from build123d import *

# Parameters (mm, degrees)
SKETCH_W        = 3.9
SKETCH_H        = 9.9
PAD_DEPTH       = 1.4
POCKET_DEPTH    = 9.901
POCKET001_DEPTH = 3.901
POCKET002_DEPTH = 0.1


with BuildPart() as part:
    # Sketch → Pad (new body)
    with BuildSketch(Plane.XY):
        Rectangle(SKETCH_W, SKETCH_H)
    extrude(amount=PAD_DEPTH)

    # Sketch001 (on Face3 of Pad) → Pocket (cut, through all)
    with BuildSketch(Plane.XZ.offset(4.95)):
        Polygon((-1.95, 0.6), (-1.65, 0), (-1.95, 0), align=None)
        Polygon((1.65, 0), (1.95, 0), (1.95, 0.6), align=None)
        Polygon((1.95, 1.4), (1.65, 1.4), (1.95, 0.8), align=None)
        Polygon((-1.95, 1.4), (-1.65, 1.4), (-1.95, 0.8), align=None)
    extrude(amount=-POCKET_DEPTH, mode=Mode.SUBTRACT)

    # Sketch002 (on Face5 of Pocket) → Pocket001 (cut, through all)
    with BuildSketch(Plane.YZ.offset(1.95)):
        Polygon((4.95, 0.8), (4.65, 1.4), (4.95, 1.4), align=None)
        Polygon((4.95, 0.6), (4.65, 0), (4.95, 0), align=None)
        Polygon((-4.95, 0.8), (-4.95, 1.4), (-4.65, 1.4), align=None)
        Polygon((-4.95, 0.6), (-4.95, 0), (-4.65, 0), align=None)
    extrude(amount=-POCKET001_DEPTH, mode=Mode.SUBTRACT)

    # Sketch003 (on Face11 of Pocket001) → Pocket002 (cut)
    with BuildSketch(Plane.XY.offset(1.4)):
        with BuildLine():
            ThreePointArc((-0.429098, 4.124211), (0, 3.695113), (0.429098, 4.124211))
            Line((0.429098, 4.124211), (0.429098, 5.299881))
            ThreePointArc((0.429098, 5.299881), (0, 5.728979), (-0.429098, 5.299881))
            Line((-0.429098, 4.124211), (-0.429098, 5.299881))
        make_face()
    extrude(amount=-POCKET002_DEPTH, mode=Mode.SUBTRACT)


with BuildPart() as part_1:
    # Body placement: moved
    add(part.part.moved(Location((0, 0, 0.1))))


solid = part_1.part
Verification items for the finished model (mm, model axes). Give positions to 0.01 mm unless a question says otherwise; leave off trailing zeros. Write each loop counter-clockwise with the first axis right and the second up, starting at its lowest first coordinate (ties: lowest second). Pieces come first, ordered by that corner, then holes. Notation, with made-up numbers: (-29, -37.5) - (-1, -37.5) arc R15 ccw to (-1, -10.5) - close; hole circle Ø5 at (19, 9.5). An arc over 180 degrees is marked (long way). Answer as CSV lines item,"result". Start each with the question number.
1. Draft check along X on faces 1 (the face through (0, 0, 1.5)), 2 (the face through (0, 4, 1.4)). Enter one of: pulls with the +X half, pulls with the -X half, needs draft (parallel to the pull), parting line crosses it, or undercut.
2. Sectioned sample at D-D (x = 1.5). Record the boundary of the cut face in (y, z), then the cut area to 3 significant figures.
3. Thickness scan on line 1 (Y direction, x = 1.25, z = 0.55) (3 decimals); line 2 (Y direction, x = -1.25, z = 1.2); line 3 (X direction, y = 1, z = 0.35) (3 decimals). Record the ranges inside material, lowest first.
4. Depth check by flat-ended pin: pin 1 (0.7 mm diameter, centred on x = 0, y = 4.5, fed in from +Z). Enter the tip coordinate at first touch or a pass-through.
5. Sectioned sample at A-A (y = -0.75). Record the boundary of the cut face in (x, z).
6. Sectioned sample at B-B (x = 0). Record the boundary of the cut face in (y, z).
7. Sectioned sample at C-C (z = 1.05). Record the boundary of the cut face in (x, y) (3 decimals).
Derived:
1,face 1,"needs draft"
1,face 2,"undercut"
2,outline,"(-4.95, 0.7) - (-4.65, 0.1) - (4.65, 0.1) - (4.95, 0.7) - (4.95, 0.9) - (4.65, 1.5) - (-4.65, 1.5) - (-4.95, 0.9) - close"
2,area,"13.5 mm²"
3,line 1,"-4.875 to 4.875"
3,line 2,"-4.8 to 4.8"
3,line 3,"-1.775 to 1.775"
4,pin 1,"z = 1.4"
5,outline,"(-1.95, 0.7) - (-1.65, 0.1) - (1.65, 0.1) - (1.95, 0.7) - (1.95, 0.9) - (1.65, 1.5) - (-1.65, 1.5) - (-1.95, 0.9) - close"
6,outline,"(-4.95, 0.7) - (-4.65, 0.1) - (4.65, 0.1) - (4.95, 0.7) - (4.95, 0.9) - (4.7, 1.4) - (3.7, 1.4) - (3.7, 1.5) - (-4.65, 1.5) - (-4.95, 0.9) - close"
7,outline,"(-1.875, -4.875) - (1.875, -4.875) - (1.875, 4.875) - (-1.875, 4.875) - close"
